```python
from build123d import *

# Parameters (mm, degrees)
SCALE1_SCALE = 0.2
SCALE2_SCALE = 1.9329
SCALE3_SCALE = 1.5


with BuildPart() as part:
    # Sketch1 → Revolve1 (revolve)
    with BuildSketch(Plane.XY, mode=Mode.PRIVATE) as revolve1_sk:
        with BuildLine():
            Line((-15.5, 37), (-8.94427191, 37))
            ThreePointArc((-8.94427191, 37), (0, 33), (8.94427191, 37))
            Line((8.94427191, 37), (15.5, 37))
            Line((15.5, 37), (15.5, 27.1))
            ThreePointArc((15.5, 27.1), (14.88492424, 25.61507576), (13.4, 25))
            Line((13.4, 25), (-13.4, 25))
            ThreePointArc((-13.4, 25), (-14.88492424, 25.61507576), (-15.5, 27.1))
            Line((-15.5, 27.1), (-15.5, 37))
        make_face()
    revolve(revolve1_sk.sketch.rotate(Axis((-31.142201835, 0, 0), (1, 0, 0)), 90), axis=Axis((-31.142201835, 0, 0), (1, 0, 0)))


with BuildPart() as part_1:
    # Scale1: scaled about (0, 0, 0)
    add(part.part.scale(SCALE1_SCALE))


with BuildPart() as part_2:
    # Scale2: scaled about (0, 0, 0)
    add(part_1.part.scale(SCALE2_SCALE))


with BuildPart() as part_3:
    # Scale3: scaled about (0, 0, 0)
    add(part_2.part.scale(SCALE3_SCALE))


solid = part_3.part
```
Check sheet for the modelled part. Datum: model origin and axes. Units: mm. Coordinates: 2 decimals unless noted, no trailing zeros. Order: outer loops, then holes, each group sorted by start corner. A loop starts at its lowest first (then second) coordinate and runs counter-clockwise, first axis right, second up. Notation, with made-up numbers: (-1, -9) -> (32, -9) arc R22 cw to (32, 24) -> close; hole circle Ø1 at (5, 20). An arc over 180 degrees is marked (long way). Write item = value, one per line. Start each with the question number.
1) Cross-section at C-C (x = 3). Enter the section's corners in (y, z).
2) Cross-section at A-A (z = 0). Enter the section's corners in (x, y), then the cut area to 3 significant figures.
3) Mould release check, pull along Y, two halves, no side actions. Record for faces 1 (the cylindrical face through (-0.109, 14.152, -3.143)), 2 (the flat face through (8.988, -11.23, -11.23)), 3 (the cylindrical face through (-7.061, -14.5, -15.813)): +Y half, -Y half, draft (parallel to the pull), parting line (faces both ways), or undercut.
4) Cross-section at D-D (x = -4). Enter the section's corners in (y, z), then the cut area to 3 significant figures.
5) Material ranges on L1, parallel to Z at x = -5, y = -11; L2, parallel to X at y = -7, z = -19; L3, parallel to Y at x = 1.5, z = -1, recorded low to high.
6) Go/stop test with flat-tipped pins: P1, Ø3, axis at x = -4.5, z = -1, coming from the -Y side; P2, Ø5, axis at y = 6.5, z = 9, coming from the +X side; P3, Ø4, axis at x = 5.5, z = -5, coming from the +Y side; P4, Ø5, axis at x = -2.5, y = 4.5, coming from the -Z side. Record where each tip stops, or that it passes through.
Ans:
q1.outline = circle Ø39.63 at (0, 0); hole circle Ø28.99 at (0, 0)
q2.outline = (-8.99, -21.46) -> (-5.19, -21.46) arc R6.96 cw to (5.19, -21.46) -> (8.99, -21.46) -> (8.99, -15.71) arc R1.22 ccw to (7.77, -14.5) -> (-7.77, -14.5) arc R1.22 ccw to (-8.99, -15.71) -> close; (-8.99, 15.71) arc R1.22 ccw to (-7.77, 14.5) -> (7.77, 14.5) arc R1.22 ccw to (8.99, 15.71) -> (8.99, 21.46) -> (5.19, 21.46) arc R6.96 cw to (-5.19, 21.46) -> (-8.99, 21.46) -> close
q2.area = 216 mm²
q3.face_1 = undercut
q3.face_2 = draft
q3.face_3 = parting line
q4.outline = circle Ø40.8 at (0, 0); hole circle Ø28.99 at (0, 0)
q4.area = 647 mm²
q5.L1 = -18.19 to -9.44, 9.44 to 18.19
q5.L2 = -8.99 to -3.77, 3.77 to 8.99
q5.L3 = -19.27 to -14.46, 14.46 to 19.27
q6.P1 = -21.46
q6.P2 = through
q6.P3 = 21.24
q6.P4 = -20.82
